Geometry check sheet. Reference: the model listing, model coordinates, mm. A direction names the side the tool comes from. Coordinates: 2 decimals unless noted, no trailing zeros. Order: outer loops, then holes, each group sorted by start corner. A loop starts at its lowest first (then second) coordinate and runs counter-clockwise, first axis right, second up.
Autodesk Fusion 360 part; units mm, degrees
sketch "Sketch1" plane through (0, 0, 0) normal (0, 1, 0) x (1, 0, 0)
  line L0 (2, 0) -> (7, 0)
  line L1 (7, 0) -> (7, -9)
  line L2 (7, -9) -> (4.7, -9)
  line L3 (4.7, -9) -> (4.7, -7.3225)
  line L4 (0, -2) -> (0, -2.6775)
  line L5 (1.2169, -4.5178) -> (3.4831, -5.4822)
  arc A0 (4.7, -7.3225) -> (3.4831, -5.4822) centre (2.7, -7.3225) ccw
  arc A1 (0, -2.6775) -> (1.2169, -4.5178) centre (2, -2.6775) ccw
  arc A2 (2, 0) -> (0, -2) centre (2, -2) ccw
  circle A3 centre (2, -2.3388) radius 1
  point P0 (4.7, -6)
  point P1 (0, -4)
  dimension "d1" = 7
  dimension "d3" = 2.3
  dimension "d4" = 3
  dimension "d5" = 4
  dimension "d6" = 2
  dimension "d7" = 2
  dimension "d8" = 2
  dimension "d10" = 2
extrude "Extrude1" add sketch "Sketch1" along normal blind 7
sketch "Sketch2" plane through (0, 0, 9) normal (0, 0, 1) x (-1, 0, 0)
  line L0 (-4.7, 0) -> (-7, 0)
  line L1 (-7, 0) -> (-7, -7)
  line L2 (-7, -7) -> (-4.7, -7)
  line L3 (-4.7, -7) -> (-4.7, 0)
  line L4 (-4.7, -7) -> (0, -7)
  line L5 (0, -7) -> (0, -5)
  line L6 (0, -5) -> (-4.7, -5)
  line L7 (-4.7, -5) -> (-4.7, -7)
  line L8 (-4.7, 0) -> (0, 0)
  line L9 (0, 0) -> (0, -2)
  line L10 (0, -2) -> (-4.7, -2)
  line L11 (-4.7, -2) -> (-4.7, 0)
  line L12 (0, -5) -> (-4.7, -5)
  line L13 (-4.7, -5) -> (-4.7, -2)
  line L14 (-4.7, -2) -> (0, -2)
  line L15 (0, -2) -> (0, -5)
extrude "Extrude2" cut sketch "Sketch2" against normal blind 10 contours L3 L6 L10 L12 L13 L14 L15
sketch "Sketch3" plane through (4.7, 0, 0) normal (-1, 0, 0) x (0, -1, 0)
  line L0 (0, 9) -> (-7, 9)
  line L1 (-7, 9) -> (-7, 7.3225)
  line L2 (-7, 7.3225) -> (-5, 7.3225)
  line L3 (-5, 7.3225) -> (-5, 0)
  line L4 (-5, 0) -> (-2, 0)
  line L5 (-2, 0) -> (-2, 7.3225)
  line L6 (-2, 7.3225) -> (0, 7.3225)
  line L7 (0, 7.3225) -> (0, 9)
  line L8 (-3.75, 7) -> (-3.25, 7)
  line L9 (-2.5, 6.25) -> (-2.5, 1.25)
  line L10 (-3.25, 0.5) -> (-3.75, 0.5)
  line L11 (-4.5, 1.25) -> (-4.5, 6.25)
  arc A0 (-3.75, 7) -> (-4.5, 6.25) centre (-3.75, 6.25) ccw
  arc A1 (-2.5, 6.25) -> (-3.25, 7) centre (-3.25, 6.25) ccw
  arc A2 (-4.5, 1.25) -> (-3.75, 0.5) centre (-3.75, 1.25) ccw
  arc A3 (-3.25, 0.5) -> (-2.5, 1.25) centre (-3.25, 1.25) ccw
  dimension "d15" = 0.75
extrude "Extrude3" cut sketch "Sketch3" against normal blind 0.2 contours L8 L9 L10 L11 A0 A1 A2 A3
fillet "Fillet1" radius 0.1 8 edges at (4.9, 3.5, 7) (4.9, 2.7197, 6.7803) (4.9, 2.5, 3.75) (4.9, 2.7197, 0.7197) (4.9, 3.5, 0.5) (4.9, 4.2803, 0.7197) (4.9, 4.5, 3.75) (4.9, 4.2803, 6.7803)
sketch "Sketch4" plane through (0, 0, 0) normal (0, -1, 0) x (1, 0, 0)
  circle A0 centre (2, 2.3388) radius 1
  line L0 (2, 0) -> (7, 0)
  line L1 (7, 0) -> (7, 9)
  line L2 (7, 9) -> (4.7, 9)
  line L3 (4.7, 9) -> (4.7, 7.3225)
  arc A1 (3.4831, 5.4822) -> (4.7, 7.3225) centre (2.7, 7.3225) ccw
  line L4 (3.4831, 5.4822) -> (1.2169, 4.5178)
  arc A2 (1.2169, 4.5178) -> (0, 2.6775) centre (2, 2.6775) ccw
  line L5 (0, 2.6775) -> (0, 2)
  arc A3 (0, 2) -> (2, 0) centre (2, 2) ccw
  line L6 (4.7, 9) -> (5.43, 9)
  line L7 (7, 9) -> (6.27, 9)
  arc A4 (5.43, 9) -> (6.27, 9) centre (5.85, 9.066) ccw
  line L8 (5.43, 9) -> (6.27, 9)
  dimension "d20" = 0.73
  dimension "d21" = 0.73
extrude "Extrude4" cut sketch "Sketch4" against normal blind 7 contours L2 A4 L8
fillet "Fillet2" radius 0.2 2 edges at (5.43, 3.5, 9) (6.27, 3.5, 9)
fillet "Fillet4" radius 1 1 edges at (7, 3.5, 0)
sketch "Sketch5" plane through (0, 0, 0) normal (0, 0, -1) x (1, 0, 0)
  line L0 (6, -7) -> (6, 0)
  line L1 (6, 0) -> (2, 0)
  line L2 (2, 0) -> (2, -2)
  line L3 (2, -2) -> (4.7, -2)
  line L4 (4.7, -2) -> (4.7, -5)
  line L5 (4.7, -5) -> (2, -5)
  line L6 (2, -5) -> (2, -7)
  line L7 (2, -7) -> (6, -7)
  line L8 (7, 0) -> (6.24, 0)
  line L9 (6.24, 0) -> (5.24, 0)
  line L10 (5.24, 0) -> (5.24, -6.5)
  line L11 (6.24, -6.5) -> (6.24, 0)
  line L12 (5.24, 0) -> (5.24, -0.5)
  line L13 (5.24, -0.5) -> (6.24, -0.5)
  line L14 (5.24, -6.5) -> (6.24, -6.5)
  dimension "d30" = 0.76
  dimension "d31" = 1
  dimension "d33" = 0.5
extrude "Extrude5" cut sketch "Sketch5" against normal blind 7 contours L0 L10 L13 L14 | L0 L11 L13 L14
fillet "Fillet5" radius 0.1 8 edges at (4.7, 3.5, 7) (4.7, 2.7197, 6.7803) (4.7, 2.5, 3.75) (4.7, 2.7197, 0.7197) (4.7, 3.5, 0.5) (4.7, 4.2803, 0.7197) (4.7, 4.5, 3.75) (4.7, 4.2803, 6.7803)
Item 1: Tool access check on faces 1 (the face through (4.36, 0.99, 6.21)), 2 (the face through (6, 0.5, 3)), 3 (the face through (4.9, 4, 4)), 4 (the face through (3, 2, 3)). Record the directions out of +Z, -Z, +X, -X, +Y, -Y that give a thin tool (end or side, any length) a straight path to the whole face; none if there is none.
Item 2: Depth check by flat-ended pin: P1, Ø1, axis at x = 6, y = 5, coming from the -Z side; P2, Ø1.8, axis at y = 4, z = 3, coming from the -X side; P3, Ø1.8, axis at x = 2, z = 2.34, coming from the +Y side. Enter the tip coordinate at first touch or a pass-through.
Item 3: Sectioned sample at A-A (x = 0.5). Record the cut outline in (y, z), and give its area (3 significant figures).
Item 4: Sectioned sample at D-D (x = 2.75). Record the cut outline in (y, z), and give its area (3 significant figures).
Item 5: Thickness scan on line 1 along X through (y, z) = (4.25, 3.75); line 2 along Y through (x, z) = (3.75, 5); line 3 along X through (y, z) = (6.25, 3). Record the ranges inside material, lowest first.
Item 6: Release check for a two-part mould opening along Y. For faces 5 (the face through (1.26, 0.99, 3.01)), 6 (the face through (4.7, 4, 8)), 7 (the face through (4, 7, 3)) record: pulls with the +Y half, pulls with the -Y half, needs draft (parallel to the pull), parting line crosses it, or undercut.
Item 7: Sectioned sample at B-B (y = 6.75). Record the cut outline in (x, z).
Geometry check:
1. face 1: +Z, -X, +Y, -Y
1. face 2: -Z
1. face 3: -X
1. face 4: +Z, -Z, -X
2. P1: stops at z = 0.03
2. P2: stops at x = 4.7
2. P3: passes through
3. outline: (0, 0.68) - (2, 0.68) - (2, 4) - (0, 4) - close; (5, 0.68) - (7, 0.68) - (7, 4) - (5, 4) - close
3. area: 13.3 mm2
4. outline: (0, 0) - (2, 0) - (2, 1.68) - (0, 1.68) - close; (0, 3) - (2, 3) - (2, 5.17) - (0, 5.17) - close; (5, 0) - (7, 0) - (7, 1.68) - (5, 1.68) - close; (5, 3) - (7, 3) - (7, 5.17) - (5, 5.17) - close
4. area: 15.4 mm2
5. line 1: x = 4.9 to 5.24, 6.24 to 7
5. line 2: y = 0 to 2, 5 to 7
5. line 3: x = 0.03 to 1.25, 2.75 to 5.24, 6.24 to 7
6. face 5: needs draft
6. face 6: undercut
6. face 7: pulls with the +Y half
7. outline: (0, 2) arc R2 ccw to (2, 0) - (6, 0) arc R1 ccw to (7, 1) - (7, 9) - (6.42, 9) arc R0.2 ccw to (6.23, 8.89) arc R0.43 cw to (5.47, 8.89) arc R0.2 ccw to (5.28, 9) - (4.7, 9) - (4.7, 7.32) arc R2 cw to (3.48, 5.48) - (1.22, 4.52) arc R2 ccw to (0, 2.68) - close; hole circle Ø2 at (2, 2.34)
